Source: CAD feature listing. Evaluate the final solid. Frame: model axes, mm. A direction names the side the tool comes from. Give positions to 0.01 mm unless a question says otherwise; leave off trailing zeros. Loops run counter-clockwise (first coordinate to the right, second up) from the corner with the lowest first, then second, coordinate; pieces in that order, holes last. Notation, with made-up numbers: M 25,17.5 L 80,17.5 A18 cw 80,28.5 Z; hole C -9.75,-27.75 d2. An arc over 180 degrees is marked long. Write item = value, one per line.
Autodesk Inventor part; units mm, degrees
ref_plane "YZ Plane" through (0, 0, 0) normal (1, 0, 0) x (0, 1, 0)
ref_plane "XZ Plane" through (0, 0, 0) normal (0, 1, 0) x (-1, 0, 0)
ref_plane "XY Plane" through (0, 0, 0) normal (0, 0, 1) x (1, 0, 0)
sketch "Boceto1" plane through (0, 0, 0) normal (0, 0, 1) x (1, 0, 0)
  line L0 (-15.5, -18.5) -> (-17.5, -18.5)
  line L1 (-17.5, -18.5) -> (-17.5, -37.5)
  line L2 (-17.5, -37.5) -> (17.5, -37.5)
  line L3 (17.5, -37.5) -> (17.5, 37.5)
  line L4 (17.5, 37.5) -> (-17.5, 37.5)
  line L5 (-17.5, 37.5) -> (-17.5, -0.5)
  line L6 (-17.5, -0.5) -> (-15.5, -0.5)
  line L7 (-15.5, -0.5) -> (-15.5, 35.5)
  line L8 (-15.5, 35.5) -> (15.5, 35.5)
  line L9 (15.5, 35.5) -> (15.5, -35.5)
  line L10 (15.5, -35.5) -> (-15.5, -35.5)
  line L11 (-15.5, -35.5) -> (-15.5, -18.5)
  line L12 (15.5, 35.5) -> (-15.5, 35.5)
  line L13 (-15.5, 35.5) -> (-15.5, -35.5)
  line L14 (-15.5, -35.5) -> (15.5, -35.5)
  line L15 (15.5, -35.5) -> (15.5, 35.5)
  line L16 (-15.3, -35.3) -> (-15.3, 35.3)
  line L17 (-15.3, 35.3) -> (15.3, 35.3)
  line L18 (15.3, 35.3) -> (15.3, -35.3)
  line L19 (15.3, -35.3) -> (-15.3, -35.3)
  line L20 (-14.1, 34.1) -> (-14.1, -34.1)
  line L21 (-14.1, -34.1) -> (14.1, -34.1)
  line L22 (14.1, -34.1) -> (14.1, 34.1)
  line L23 (14.1, 34.1) -> (-14.1, 34.1)
  line L24 (-15.5, -0.5) -> (-14.1, -0.5)
  line L25 (-15.5, -18.5) -> (-14.1, -18.5)
  point P0 (0, 0)
  point P1 (-15.3, -0.5)
  point P2 (-15.3, -18.5)
  dimension "d0" = 0.2
  dimension "d1" = 1.2
extrude "Extrusión1" add sketch "Boceto1" against normal blind 3 contours L25 L20 L21 L22 L23 L24 L16 L17 L18 L19
chamfer "Chaflán1" distance 0.8 angle 45 5 edges at (-15.3, 17.4, -3) (-15.3, -26.9, -3) (0, -35.3, -3) (15.3, 0, -3) (0, 35.3, -3)
sketch "Boceto2" plane through (0, 0, 0) normal (0, 0, 1) x (1, 0, 0)
  line L0 (-15.5, -18.5) -> (-17.5, -18.5)
  line L1 (-17.5, -18.5) -> (-17.5, -37.5)
  line L2 (-17.5, -37.5) -> (17.5, -37.5)
  line L3 (17.5, -37.5) -> (17.5, 37.5)
  line L4 (17.5, 37.5) -> (-17.5, 37.5)
  line L5 (-17.5, 37.5) -> (-17.5, -0.5)
  line L6 (-17.5, -0.5) -> (-15.5, -0.5)
  line L7 (-15.5, -0.5) -> (-15.5, 35.5)
  line L8 (-15.5, 35.5) -> (15.5, 35.5)
  line L9 (15.5, 35.5) -> (15.5, -35.5)
  line L10 (15.5, -35.5) -> (-15.5, -35.5)
  line L11 (-15.5, -35.5) -> (-15.5, -18.5)
  line L12 (-17.5, -0.5) -> (-17.5, -18.5)
  point P0 (0, 0)
extrude "Extrusión2" add sketch "Boceto2" along normal blind 1.5
sketch "Boceto3" plane through (0, 0, 1.5) normal (0, 0, 1) x (1, 0, 0)
  line L0 (-17.5, 37.5) -> (-17.5, -37.5)
  line L1 (-17.5, -37.5) -> (17.5, -37.5)
  line L2 (17.5, -37.5) -> (17.5, 37.5)
  line L3 (17.5, 37.5) -> (-17.5, 37.5)
  line L4 (-15.5, 35.5) -> (15.5, 35.5)
  line L5 (-15.5, -35.5) -> (-15.5, 35.5)
  line L6 (15.5, -35.5) -> (-15.5, -35.5)
  line L7 (15.5, 35.5) -> (15.5, -35.5)
  line L8 (-15.5, 35.5) -> (-15.5, 15.5)
  line L9 (-15.5, 15.5) -> (-0.5, 15.5)
  line L10 (-0.5, 15.5) -> (-15.5, 15.5)
  line L11 (-15.5, 15.5) -> (-15.5, 0.5)
  line L12 (-15.5, 0.5) -> (-0.5, 0.5)
  line L13 (-0.5, 0.5) -> (-0.5, 15.5)
  circle A0 centre (-8, 8) radius 7.5
  point P0 (0, 0)
  dimension "d9" = 20
  dimension "d11" = 15
  dimension "d12" = 15
  dimension "d13" = 15
extrude "Extrusión3" cut sketch "Boceto3" against normal through all contours A0
properties part number "Tapa"
1. Pull-direction query (Y, two-part tool) for faces 1 (the flat face through (0, 37.5, 1)), 2 (the flat face through (0, -37.5, 1)), 3 (the flat face through (0, 34.1, -1)); classes: +Y half, -Y half, draft (parallel to the pull), parting line (faces both ways), or undercut.
Derived:
face_1 = +Y half
face_2 = -Y half
face_3 = undercut
2. Cut plane D-D, the plane x = 12.5. Return the cut outline in (y, z).
Derived:
outline = M -37.5,0 L -35.3,0 L -35.3,-2.2 L -34.5,-3 L -34.1,-3 L -34.1,0 L 34.1,0 L 34.1,-3 L 34.5,-3 L 35.3,-2.2 L 35.3,0 L 37.5,0 L 37.5,1.5 L -37.5,1.5 Z
3. Cut plane C-C, the plane z = -0.75. Return the cut outline in (x, y), then the cut area to 3 significant figures.
Derived:
outline = M -15.3,-35.3 L 15.3,-35.3 L 15.3,35.3 L -15.3,35.3 L -15.3,9.72 A7.5 cw -14.1,12.36 L -14.1,34.1 L 14.1,34.1 L 14.1,-34.1 L -14.1,-34.1 L -14.1,-18.5 L -15.3,-18.5 Z; M -15.3,-0.5 L -14.1,-0.5 L -14.1,3.64 A7.5 cw -15.3,6.28 Z
area = 208 mm²
4. Material intervals for probe 1 along Y at (x, z) = (-8, -1.65); probe 2 along X at (y, z) = (-32, -0.2); probe 3 along X at (y, z) = (8, 0.2), sorted ascending. Write a range as from..to.
Derived:
probe_1 = -35.3..-34.1, 34.1..35.3
probe_2 = -15.3..-14.1, 14.1..15.3
probe_3 = -17.5..-15.5, -0.5..17.5
5. Cut plane A-A, the plane x = -8. Return the cut outline in (y, z).
Derived:
outline = M -37.5,0 L -35.3,0 L -35.3,-2.2 L -34.5,-3 L -34.1,-3 L -34.1,0 L 0.5,0 L 0.5,1.5 L -37.5,1.5 Z; M 15.5,0 L 34.1,0 L 34.1,-3 L 34.5,-3 L 35.3,-2.2 L 35.3,0 L 37.5,0 L 37.5,1.5 L 15.5,1.5 Z
6. First-contact query: pin 1 Ø2.5 at (x, z) = (1, -1) entering from +Y; pin 2 Ø17.5 at (x, y) = (-3, 7.5) entering from -Z; pin 3 Ø1.5 at (y, z) = (2.5, -2) entering from +X; pin 4 Ø1.1 at (y, z) = (26.5, -1) entering from -X. Flat tips, straight axial feed; report the tip coordinate or a pass-through.
Derived:
pin_1 = 37.5
pin_2 = 0
pin_3 = 15.3
pin_4 = -15.3
7. Cut plane B-B, the plane y = 8. Return the cut outline in (x, z).
Derived:
outline = M -17.5,0 L -15.5,0 L -15.5,1.5 L -17.5,1.5 Z; M -0.5,0 L 14.1,0 L 14.1,-3 L 14.5,-3 L 15.3,-2.2 L 15.3,0 L 17.5,0 L 17.5,1.5 L -0.5,1.5 Z
8. Reachability of faces 4 (the flat face through (-14.1, 23, -1)), 5 (the flat face through (0, 35.3, -1)), 6 (the flat face through (0, -35.3, -1)), 7 (the flat face through (-15.3, 3, -1)) from +Z, -Z, +X, -X, +Y, -Y: full face, straight path, thin tool, end or side. Return the list, or none.
Derived:
face_4 = -Z
face_5 = -Z, +X, -X, +Y
face_6 = -Z, +X, -X, -Y
face_7 = -Z, -X, +Y, -Y
